Can you work these out from the model? Positions are in its coordinate system, mm. Face numbers are marked on the shaded views. A direction names the side the tool comes from. Round coordinates to 2 decimals unless told otherwise and drop trailing zeros. Loops run counter-clockwise (first coordinate to the right, second up) from the corner with the lowest first, then second, coordinate; pieces in that order, holes last. Notation, with made-up numbers: (51.25, 8) -> (99.25, 8) arc R16 ccw to (99.25, 38) -> close; hole circle Ø8 at (64.25, 20). An arc over 180 degrees is marked (long way). Write each question's results on one line, items separated by ' | '.
from build123d import *

# Parameters (mm, degrees)
F0_R     = 6
F1_DEPTH = 4.5
F2_R     = 7
F2_R_2   = 2
F3_DEPTH = 8
F4_R     = 1.5
F5_DEPTH = 3
F6_R     = 1
F7_DEPTH = 4


with BuildPart() as f1:
    # F0 (on Front) → F1 (new body, symmetric)
    with BuildSketch(Plane.XZ):
        with BuildLine():
            ThreePointArc((-8, 0), (0, -8), (8, 0))
            ThreePointArc((8, 0), (0, 8), (-8, 0))
        make_face()
        Circle(F0_R, mode=Mode.SUBTRACT)
    extrude(amount=F1_DEPTH, both=True)

    # F2 (on face) → F3 (join)
    with BuildSketch(Plane(origin=(0, 4.5, 0), x_dir=(-1, 0, 0), z_dir=(0, 1, 0))):
        Circle(F2_R)
        Circle(F2_R_2, mode=Mode.SUBTRACT)
    extrude(amount=F3_DEPTH)

    # F4 (on Right) → F5 (join, symmetric)
    with BuildSketch(Plane.YZ):
        with BuildLine():
            Line((4.5, 8), (-5.5923303169, 16.3153393661))
            ThreePointArc((-5.5923303169, 16.3153393661), (-9.8582842332, 15.8543180621), (-9.3, 11.6))
            Line((-9.3, 11.6), (-4.5, 8))
            Line((-4.5, 8), (-4.5, 6))
            Line((-4.5, 6), (4.5, 6))
            Line((4.5, 6), (4.5, 8))
        make_face()
        with Locations((-7.5, 14)):
            Circle(F4_R, mode=Mode.SUBTRACT)
    extrude(amount=F5_DEPTH, both=True)

    # F6 (on Right) → F7 (join, symmetric)
    with BuildSketch(Plane.YZ):
        with BuildLine():
            Line((-4.5, -6), (-4.5, -7.7087121525))
            ThreePointArc((-4.5, -7.7087121525), (-5.3825642408, -11.6449777747), (-1.3635014837, -11.2982195846))
            ThreePointArc((-1.3635014837, -11.2982195846), (1.1362631614, -8.8811345092), (4.5, -8))
            Line((4.5, -8), (4.5, -6))
            Line((4.5, -6), (-4.5, -6))
        make_face()
        with Locations((-3.5, -10)):
            Circle(F6_R, mode=Mode.SUBTRACT)
    extrude(amount=F7_DEPTH, both=True)


solid = f1.part
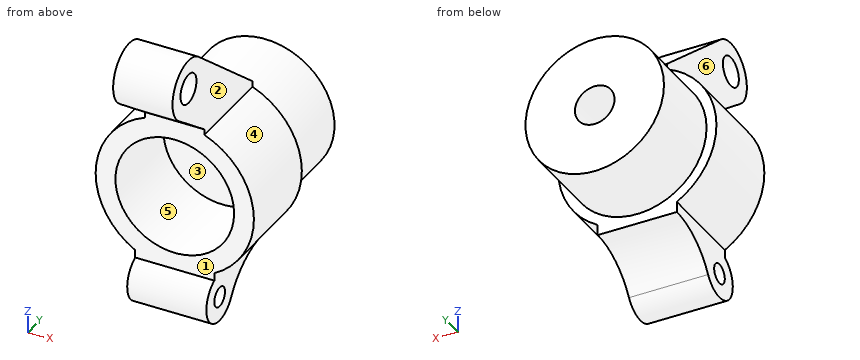
1. We'd pull the mould along Z, two halves only. Please class the marked faces 4, 5 and 6: pulls with the +Z half, pulls with the -Z half, needs draft (parallel to the pull), parting line crosses it, or undercut.
Final values:
face 4: parting line crosses it | face 5: undercut | face 6: needs draft
2. If we section it at A-A (x = 0): List the corners of the cut face in (y, z) for me, then the cut area to 3 significant figures.
Final values:
outline: (-9.3, 11.6) -> (-4.5, 8) -> (-4.5, 6) -> (4.5, 6) -> (4.5, 2) -> (12.5, 2) -> (12.5, 7) -> (4.5, 7) -> (4.5, 8) -> (-5.59, 16.32) arc R3 ccw (long way) to start; (-4.5, -7.71) arc R2.5 ccw (long way) to (-1.36, -11.3) arc R6.86 cw to (4.5, -8) -> (4.5, -7) -> (12.5, -7) -> (12.5, -2) -> (4.5, -2) -> (4.5, -6) -> (-4.5, -6) -> close; hole circle Ø3 at (-7.5, 14); hole circle Ø2 at (-3.5, -10) | area: 200 mm2
3. Will these pins go through, and if not, where does the flat tip stop? pin 1 (5 mm diameter, centred on y = -6.5, z = 10, fed in from +X); pin 2 (1 mm diameter, centred on y = 4, z = -8, fed in from -X); pin 3 (5 mm diameter, centred on y = -4, z = 13, fed in from -X).
Final values:
pin 1: x = 3 | pin 2: x = -4 | pin 3: x = -3
4. On a 3-axis mill with a long thin cutter (end or side, diameter ignored), from which of +Z, -Z, +X, -X, +Y, -Y can I reach the whole of each face in a straight line? I mean the marked faces 1, 2 and 3. Say none if no direction works.
Final values:
face 1: +X, -X, -Y | face 2: +Z, +X, +Y, -Y | face 3: -Y
5. If we section it at B-B (y = -7.5): List the corners of the cut face in (x, z) for me.
Final values:
outline: (-3, 10.25) -> (3, 10.25) -> (3, 12.5) -> (-3, 12.5) -> close; (-3, 15.5) -> (3, 15.5) -> (3, 17) -> (-3, 17) -> close
6. If we section it at D-D (x = 3.5): List the corners of the cut face in (y, z) for me, then the cut area to 3 significant figures.
Final values:
outline: (-4.5, -7.71) arc R2.5 ccw (long way) to (-1.36, -11.3) arc R6.86 cw to (4.5, -8) -> (4.5, -6.06) -> (12.5, -6.06) -> (12.5, 6.06) -> (4.5, 6.06) -> (4.5, 7.19) -> (-4.5, 7.19) -> (-4.5, 4.87) -> (4.5, 4.87) -> (4.5, -4.87) -> (-4.5, -4.87) -> close; hole circle Ø2 at (-3.5, -10) | area: 167 mm2
7. Please list where these lines run through material, in increasing order: line 1 (Z direction, x = 2.5, y = -2.75); line 2 (Z direction, x = 1, y = -3.5); line 3 (Z direction, x = 2, y = 1.25). Write a range as from..to.
Final values:
line 1: -12.38..-10.66, -9.34..-5.45, 5.45..13.97 | line 2: -12.5..-11, -9..-5.92, 5.92..14.59 | line 3: -8.82..-5.66, 5.66..10.68
8. If we section it at C-C (y = -3.5): List the corners of the cut face in (x, z) for me.
Final values:
outline: (-4, -12.5) -> (4, -12.5) -> (4, -11) -> (-4, -11) -> close; (-4, -9) -> (4, -9) -> (4, -6.93) arc R8 ccw to (3, 7.42) -> (3, 14.59) -> (-3, 14.59) -> (-3, 7.42) arc R8 ccw to (-4, -6.93) -> close; hole circle Ø12 at (0, 0)
